```python
from build123d import *

# Parameters (mm, degrees)
F1_DEPTH = 142.875
F3_DEPTH = 1.00176


with BuildPart() as f1:
    # F0 (on Front) → F1 (new body, symmetric)
    with BuildSketch(Plane.XZ):
        with BuildLine():
            ThreePointArc((-13.5001, 1.99898), (-12.914612, 0.585488), (-11.50112, 0))
            Line((-11.50112, 0), (11.50112, 0))
            ThreePointArc((11.50112, 0), (12.914612, 0.585488), (13.5001, 1.99898))
            Line((13.5001, 1.99898), (13.5001, 5.4991))
            ThreePointArc((13.5001, 5.4991), (13.793216, 6.206744), (14.50086, 6.49986))
            Line((14.50086, 6.49986), (18.328109, 6.49986))
            Line((18.328109, 6.49986), (18.328109, 7.50062))
            Line((18.328109, 7.50062), (14.5161, 7.50062))
            ThreePointArc((14.5161, 7.50062), (13.102608, 6.915132), (12.51712, 5.50164))
            Line((12.51712, 5.50164), (12.51712, 2.00152))
            ThreePointArc((12.51712, 2.00152), (12.224004, 1.293876), (11.51636, 1.00076))
            Line((11.51636, 1.00076), (-11.48334, 1.00076))
            ThreePointArc((-11.48334, 1.00076), (-12.190984, 1.293876), (-12.4841, 2.00152))
            Line((-12.4841, 2.00152), (-12.4841, 5.50164))
            ThreePointArc((-12.4841, 5.50164), (-13.069588, 6.915132), (-14.48308, 7.50062))
            Line((-14.48308, 7.50062), (-16.673091, 7.50062))
            Line((-16.673091, 7.50062), (-16.673091, 6.49986))
            Line((-16.673091, 6.49986), (-14.50086, 6.49986))
            ThreePointArc((-14.50086, 6.49986), (-13.793216, 6.206744), (-13.5001, 5.4991))
            Line((-13.5001, 5.4991), (-13.5001, 1.99898))
        make_face()
    extrude(amount=F1_DEPTH, both=True)

    # F2 (on face) → F3 (cut, through all)
    with BuildSketch(Plane.XY.offset(1.00076)):
        with BuildLine():
            ThreePointArc((2.59969, 29.69895), (0, 32.29864), (-2.59969, 29.69895))
            Line((-2.59969, 29.69895), (-2.59969, 9.89965))
            ThreePointArc((-2.59969, 9.89965), (0, 7.29996), (2.59969, 9.89965))
            Line((2.59969, 9.89965), (2.59969, 29.69895))
        make_face()
        with BuildLine():
            ThreePointArc((-2.59969, 45.89907), (0, 43.29938), (2.59969, 45.89907))
            Line((2.59969, 45.89907), (2.59969, 65.69837))
            ThreePointArc((2.59969, 65.69837), (0, 68.29806), (-2.59969, 65.69837))
            Line((-2.59969, 65.69837), (-2.59969, 45.89907))
        make_face()
        with BuildLine():
            ThreePointArc((-2.59969, 81.89849), (0, 79.2988), (2.59969, 81.89849))
            Line((2.59969, 81.89849), (2.59969, 101.69779))
            ThreePointArc((2.59969, 101.69779), (0, 104.29748), (-2.59969, 101.69779))
            Line((-2.59969, 101.69779), (-2.59969, 81.89849))
        make_face()
        with BuildLine():
            ThreePointArc((-2.59969, 117.89791), (0, 115.29822), (2.59969, 117.89791))
            Line((2.59969, 117.89791), (2.59969, 137.69721))
            ThreePointArc((2.59969, 137.69721), (0, 140.2969), (-2.59969, 137.69721))
            Line((-2.59969, 137.69721), (-2.59969, 117.89791))
        make_face()
        with BuildLine():
            ThreePointArc((-2.59969, -26.09977), (0, -28.69946), (2.59969, -26.09977))
            Line((2.59969, -26.09977), (2.59969, -6.30047))
            ThreePointArc((2.59969, -6.30047), (0, -3.70078), (-2.59969, -6.30047))
            Line((-2.59969, -6.30047), (-2.59969, -26.09977))
        make_face()
        with BuildLine():
            ThreePointArc((-2.59969, -62.09919), (0, -64.69888), (2.59969, -62.09919))
            Line((2.59969, -62.09919), (2.59969, -42.29989))
            ThreePointArc((2.59969, -42.29989), (0, -39.7002), (-2.59969, -42.29989))
            Line((-2.59969, -42.29989), (-2.59969, -62.09919))
        make_face()
        with BuildLine():
            ThreePointArc((-2.59969, -98.09861), (0, -100.6983), (2.59969, -98.09861))
            Line((2.59969, -98.09861), (2.59969, -78.29931))
            ThreePointArc((2.59969, -78.29931), (0, -75.69962), (-2.59969, -78.29931))
            Line((-2.59969, -78.29931), (-2.59969, -98.09861))
        make_face()
        with BuildLine():
            ThreePointArc((-2.59969, -134.10311), (0, -136.7028), (2.59969, -134.10311))
            Line((2.59969, -134.10311), (2.59969, -114.30381))
            ThreePointArc((2.59969, -114.30381), (0, -111.70412), (-2.59969, -114.30381))
            Line((-2.59969, -114.30381), (-2.59969, -134.10311))
        make_face()
    extrude(amount=-F3_DEPTH, mode=Mode.SUBTRACT)


solid = f1.part
```
Can you work these out from the model? Positions are in its coordinate system, mm. Round coordinates to 2 decimals unless told otherwise and drop trailing zeros. Loops run counter-clockwise (first coordinate to the right, second up) from the corner with the lowest first, then second, coordinate; pieces in that order, holes last. Notation, with made-up numbers: (18, 14.25) -> (41, 14.25) arc R17 ccw to (41, 23.25) -> close; hole circle Ø11 at (41.25, -39). An arc over 180 degrees is marked (long way). Answer in a Markdown table with one row per item.
Item 1: Suppose I cut it at C-C, the plane y = -106. List the corners of the cut face in (x, z) for me, plus the area to 3 significant figures.
Answer block:
| item | result |
|---|---|
| outline | (-16.67, 6.5) -> (-14.5, 6.5) arc R1 cw to (-13.5, 5.5) -> (-13.5, 2) arc R2 ccw to (-11.5, 0) -> (11.5, 0) arc R2 ccw to (13.5, 2) -> (13.5, 5.5) arc R1 cw to (14.5, 6.5) -> (18.33, 6.5) -> (18.33, 7.5) -> (14.52, 7.5) arc R2 ccw to (12.52, 5.5) -> (12.52, 2) arc R1 cw to (11.52, 1) -> (-11.48, 1) arc R1 cw to (-12.48, 2) -> (-12.48, 5.5) arc R2 ccw to (-14.48, 7.5) -> (-16.67, 7.5) -> close |
| area | 45.5 mm² |
Item 2: We'd pull the mould along X, two halves only. Please class faces 1 (the flat face through (0, -2, 1.001)), 2 (the flat face through (0.7, -142.875, 0.7)): released by +X, released by -X, zero draft, split by the parting line, or undercut.
Answer block:
| item | result |
|---|---|
| face 1 | undercut |
| face 2 | zero draft |
Item 3: Will these pins go through, and if not, where does the flat tip stop? P1, Ø18.5, axis at x = 3, y = 30.5, coming from the +Z side; P2, Ø1.1, axis at y = 13, z = 3, coming from the -X side; P3, Ø4, axis at x = 16.5, y = 47, coming from the -Z side.
Answer block:
| item | result |
|---|---|
| P1 | z = 1.32 |
| P2 | x = -13.5 |
| P3 | z = 6.5 |
Item 4: Suppose I cut it at B-B, the plane x = 0. Give the number of separate pieces and of enclosed holes in the cut face, plus the area to 3 significant figures.
Answer block:
| item | result |
|---|---|
| separate pieces | 9 |
| enclosed holes | 0 |
| area | 85.8 mm² |
Item 5: Suppose I cut it at A-A, the plane y = 12.5. List the corners of the cut face in (x, z) for me, plus the area to 3 significant figures.
Answer block:
| item | result |
|---|---|
| outline | (-16.67, 6.5) -> (-14.5, 6.5) arc R1 cw to (-13.5, 5.5) -> (-13.5, 2) arc R2 ccw to (-11.5, 0) -> (-2.6, 0) -> (-2.6, 1) -> (-11.48, 1) arc R1 cw to (-12.48, 2) -> (-12.48, 5.5) arc R2 ccw to (-14.48, 7.5) -> (-16.67, 7.5) -> close; (2.6, 0) -> (11.5, 0) arc R2 ccw to (13.5, 2) -> (13.5, 5.5) arc R1 cw to (14.5, 6.5) -> (18.33, 6.5) -> (18.33, 7.5) -> (14.52, 7.5) arc R2 ccw to (12.52, 5.5) -> (12.52, 2) arc R1 cw to (11.52, 1) -> (2.6, 1) -> close |
| area | 40.2 mm² |
Item 6: If I drill on probe 1 along X at (y, z) = (-1.5, 1.75) (3 decimals); probe 2 along Z at (x, y) = (8, -130); probe 3 along Z at (x, y) = (15.5, 50), over which ranges is the centre line in solid material (lowest first)?
Answer block:
| item | result |
|---|---|
| probe 1 | -13.485 to -12.452, 12.485 to 13.485 |
| probe 2 | 0 to 1 |
| probe 3 | 6.5 to 7.5 |
